Could you check a few things on this model? Use its own coordinates, in mm. A direction names the side the tool comes from. Give positions to 0.01 mm unless a question says otherwise; leave off trailing zeros. Loops run counter-clockwise (first coordinate to the right, second up) from the corner with the lowest first, then second, coordinate; pieces in that order, holes last. Notation, with made-up numbers: M -4.5,-17.5 L 11.5,-17.5 A10 ccw 11.5,-11.5 Z; hole C 70,50 d7. An arc over 180 degrees is marked long. Return JSON: item names as keys, results as strings. Group by question number.
1. If we section it at A-A (z = -80): Write out the boundary of the cut face in (x, y), plus the area to 3 significant figures.
2. If we section it at C-C (x = 131.5): Write out the boundary of the cut face in (y, z).
3. For pin 1 (4 mm diameter, centred on x = 17, y = 3.5, fed in from -Z); pin 2 (6.5 mm diameter, centred on x = 124, y = 5.5, fed in from -Z); pin 3 (4 mm diameter, centred on x = 208, y = 8.5, fed in from +Z), each with a flat end and sliding along its axis, tell me the tip position at first contact or that it passes through.
4. If we section it at D-D (z = -413): Write out the boundary of the cut face in (x, y).
5. Please list where these lines run through material, in increasing order: line 1 (X direction, y = 7.75, z = -61.5); line 2 (Z direction, x = 128, y = 10.5); line 3 (Z direction, x = 279, y = 2).
6. If we section it at B-B (y = 9.5): Write out the boundary of the cut face in (x, z), plus the area to 3 significant figures.
7. If we mould it in two halves opening along X, with no side actions, what happens to faces 1 (the flat face through (304.8, 6, -169)), 2 (the flat face through (49, 0, -176)), 3 (the cylindrical face through (236.029, 6.261, -400.432)), 4 (the cylindrical face through (69.509, 6.261, -398.958))? For each: +X half, -X half, draft (parallel to the pull), parting line (faces both ways), or undercut.
8. For faces 5 (the flat face through (153, 6, -50.8)), 6 (the flat face through (0, 6, -174)), 7 (the flat face through (150, 6, 0)), 8 (the flat face through (289, 6, -342.9)), 9 (the flat face through (31.75, 6, -394)), which set-ups out of +Z, -Z, +X, -X, +Y, -Y let a thin tool reach every point of the face, with its end or its side?
```python
from build123d import *

# Parameters (mm, degrees)
BOSS_EXTRUDE1_DEPTH = 12.7


with BuildPart() as part:
    # Sketch2 → Boss-Extrude1 (new body)
    with BuildSketch(Plane(origin=(0, 0, 0), x_dir=(1, 0, 0), z_dir=(0, 1, 0))):
        with BuildLine():
            Line((0, 0), (304.8, 0))
            Line((304.8, 0), (304.8, 342.9))
            Line((304.8, 342.9), (273.05, 342.9))
            Line((273.05, 342.9), (273.05, 444.5))
            ThreePointArc((273.05, 444.5), (235.657746743, 399.696126628), (222.25, 342.9))
            Line((222.25, 342.9), (222.25, 50.8))
            Line((222.25, 50.8), (82.55, 50.8))
            Line((82.55, 50.8), (82.55, 342.9))
            ThreePointArc((82.55, 342.9), (69.142253257, 399.696126628), (31.75, 444.5))
            Line((31.75, 444.5), (31.75, 342.9))
            Line((31.75, 342.9), (0, 342.9))
            Line((0, 342.9), (0, 0))
        make_face()
    extrude(amount=BOSS_EXTRUDE1_DEPTH)


solid = part.part
```
Answer:
{
 "1": {"outline": "M 0,0 L 82.55,0 L 82.55,12.7 L 0,12.7 Z; M 222.25,0 L 304.8,0 L 304.8,12.7 L 222.25,12.7 Z", "area": "2,100 mm²"},
 "2": {"outline": "M 0,-50.8 L 12.7,-50.8 L 12.7,0 L 0,0 Z"},
 "3": {"pin 1": "stops at z = -342.9", "pin 2": "stops at z = -50.8", "pin 3": "stops at z = 0"},
 "4": {"outline": "M 31.75,0 L 61.45,0 L 61.45,12.7 L 31.75,12.7 Z; M 243.35,0 L 273.05,0 L 273.05,12.7 L 243.35,12.7 Z"},
 "5": {"line 1": "x = 0 to 82.55, 222.25 to 304.8", "line 2": "z = -50.8 to 0", "line 3": "z = -342.9 to 0"},
 "6": {"outline": "M 0,-342.9 L 31.75,-342.9 L 31.75,-444.5 A127 ccw 82.55,-342.9 L 82.55,-50.8 L 222.25,-50.8 L 222.25,-342.9 A127 ccw 273.05,-444.5 L 273.05,-342.9 L 304.8,-342.9 L 304.8,0 L 0,0 Z", "area": "70,900 mm²"},
 "7": {"face 1": "+X half", "face 2": "draft", "face 3": "undercut", "face 4": "undercut"},
 "8": {"face 5": "-Z, +Y, -Y", "face 6": "+Z, -Z, -X, +Y, -Y", "face 7": "+Z, +X, -X, +Y, -Y", "face 8": "-Z, +X, +Y, -Y", "face 9": "-Z, -X, +Y, -Y"}
}
